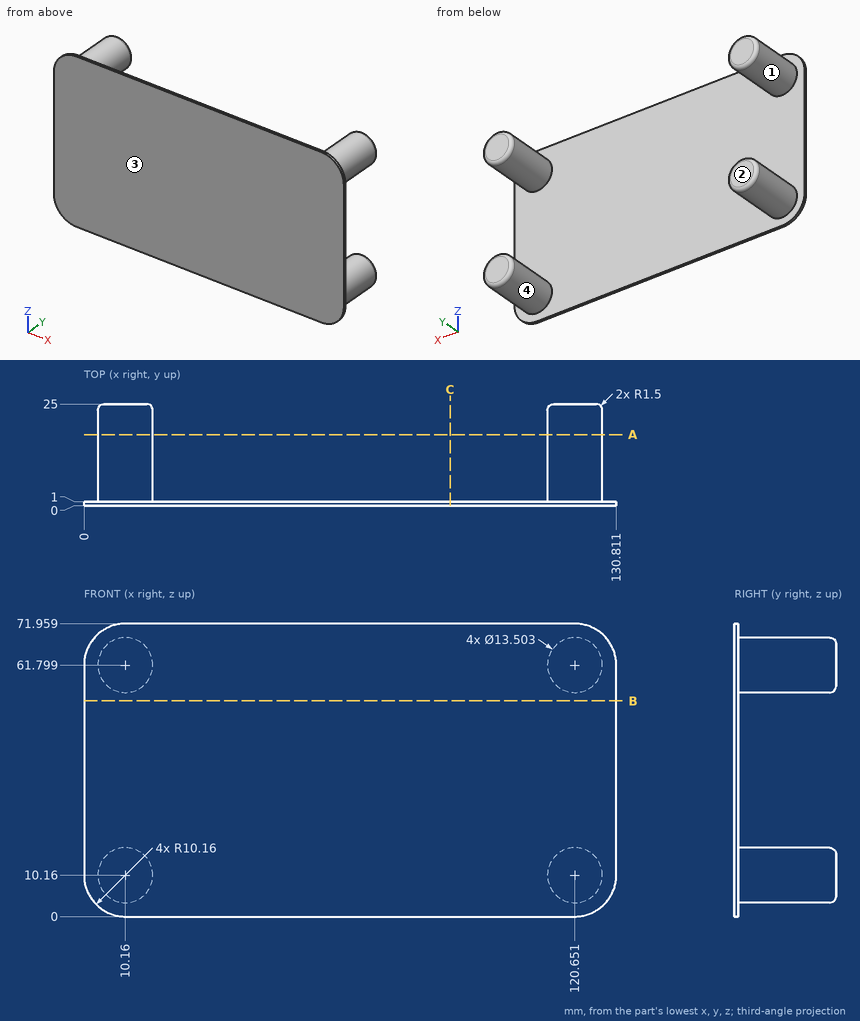
The drawing under review shows one solid part. Ordinate dimensions are in mm from its lowest x, y, z. A direction names the side the tool comes from. Give positions to 0.01 mm unless a question says otherwise; leave off trailing zeros. Write each loop counter-clockwise with the first axis right and the second up, starting at its lowest first coordinate (ties: lowest second). Pieces come first, ordered by that corner, then holes.
1. Draft analysis for pull direction X (two halves, no side actions). For the marked faces 1 and 2, state which applies: +X half, -X half, draft (parallel to the pull), parting line (faces both ways), or undercut.
2. Tool access review of the marked faces 3 and 4: name each direction out of +Z, -Z, +X, -X, +Y, -Y from which nothing blocks a thin tool from reaching the whole face with its end or side.
3. For P1, Ø3, axis at x = 34, z = 44, coming from the +Y side, flat-tipped, find the tip position at first contact; note if it passes through.
4. Add section A-A, the plane y = 17.5. Write out the cut boundary in (x, z), plus the area to 3 significant figures.
5. Wall thickness on L1, parallel to Y at x = 52.5, z = 20.5; L2, parallel to X at y = 7.25, z = 56.5 (1 decimal); L3, parallel to Z at x = 6, y = 13: over which ranges is each line inside the solid? List them lowest first.
6. Add section C-C, the plane x = 90. Write out the cut boundary in (y, z).
7. Add section B-B, the plane z = 53. Write out the cut boundary in (x, y).
Worked answers:
1. face 1: undercut
1. face 2: draft
2. face 3: +Z, -Z, +X, -X, -Y
2. face 4: +Y
3. P1: stops at y = 1
4. outline: circle Ø13.5 at (10.16, 10.16); circle Ø13.5 at (10.16, 61.8); circle Ø13.5 at (120.65, 10.16); circle Ø13.5 at (120.65, 61.8)
4. area: 573 mm2
5. L1: y = 0 to 1
5. L2: x = 6 to 14.3, 116.5 to 124.8
5. L3: z = 4.84 to 15.48, 56.48 to 67.12
6. outline: (0, 0) - (1, 0) - (1, 71.96) - (0, 71.96) - close
7. outline: (0, 0) - (130.81, 0) - (130.81, 1) - (0, 1) - close
